Read the model definition and answer for the solid it produces. Units are mm, in the model's axes. Face numbers are marked on the shaded views. A direction names the side the tool comes from. Coordinates: 2 decimals unless noted, no trailing zeros. Write each loop counter-clockwise with the first axis right and the second up, starting at its lowest first coordinate (ties: lowest second). Pieces come first, ordered by that corner, then holes.
(1) Find the intervals of material crossed by probe 1 along Z at (x, y) = (-47.5, -14.5); probe 2 along Z at (x, y) = (-7, -13.5); probe 3 along X at (y, z) = (-8.75, 15), in increasing order.
(2) Which of the six approach directions +Z, -Z, +X, -X, +Y, -Y give full straight-line access (tool end or side, diameter ignored) to the marked faces 5 and 6?
(3) Given pin 1 (6 mm diameter, centred on y = -20.5, z = -2.5, fed in from -X); pin 2 (1 mm diameter, centred on y = -7, z = 52, fed in from +X); pin 3 (1 mm diameter, centred on y = -3.5, z = 47.5, fed in from +X), each flat-ended and moving along its own axis, determine where each tip first touches the part or whether it passes through.
(4) The mould has two halves that part along Z. Classify the marked faces 1, 2, 3 and 4: +Z half, -Z half, draft (parallel to the pull), parting line (faces both ways), or undercut.
(5) Section B-B on y = -13.5 is taken. Write down the section's boundary in (x, z), then the cut area to 3 significant figures.
(6) Section A-A on x = -51.5 is taken. Write down the section's boundary in (y, z), then the cut area to 3 significant figures.
(7) Section D-D on z = 28 is taken. Write down the section's boundary in (x, y).
(8) Section C-C on x = -22.5 is taken. Write down the section's boundary in (y, z).
from build123d import *

# Parameters (mm, degrees)
F1_DEPTH = 25.4


with BuildPart() as f1:
    # F0 (on Front) → F1 (new body)
    with BuildSketch(Plane.XZ):
        with BuildLine():
            Line((6.587991, 76.630748), (-56.699019, 76.630748))
            Line((-56.699019, 76.630748), (-56.699019, 33.66233))
            Line((-56.699019, 33.66233), (-44.595942, 33.66233))
            Line((-44.595942, 33.66233), (-44.595942, -7.400833))
            Line((-44.595942, -7.400833), (-56.699019, -7.400833))
            Line((-56.699019, -7.400833), (-56.699019, -50.369252))
            Line((-56.699019, -50.369252), (6.587991, -50.369252))
            Line((6.587991, -50.369252), (6.587991, -31.048073))
            ThreePointArc((6.587991, -31.048073), (-37.59083, 13.130748), (6.587991, 57.30957))
            Line((6.587991, 57.30957), (6.587991, 76.630748))
        make_face()
    extrude(amount=F1_DEPTH)


solid = f1.part
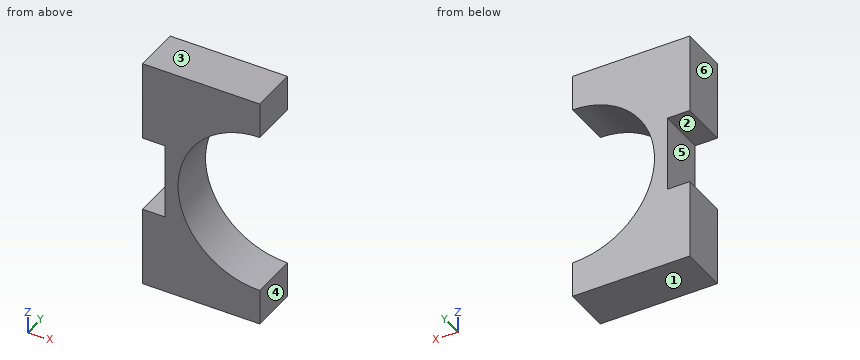
Response:
1. probe 1: z = -50.37 to -7.4, 33.66 to 76.63
1. probe 2: z = -50.37 to -28.91, 55.17 to 76.63
1. probe 3: x = -44.6 to -37.55
2. face 5: -X, +Y, -Y
2. face 6: +Z, -Z, -X, +Y, -Y
3. pin 1: stops at x = -44.6
3. pin 2: stops at x = -13.46
3. pin 3: stops at x = -20.54
4. face 1: -Z half
4. face 2: undercut
4. face 3: +Z half
4. face 4: draft
5. outline: (-56.7, -50.37) - (6.59, -50.37) - (6.59, -31.05) arc R44.18 cw to (6.59, 57.31) - (6.59, 76.63) - (-56.7, 76.63) - (-56.7, 33.66) - (-44.6, 33.66) - (-44.6, -7.4) - (-56.7, -7.4) - close
5. area: 4,470 mm2
6. outline: (-25.4, -50.37) - (0, -50.37) - (0, -7.4) - (-25.4, -7.4) - close; (-25.4, 33.66) - (0, 33.66) - (0, 76.63) - (-25.4, 76.63) - close
6. area: 2,180 mm2
7. outline: (-44.6, -25.4) - (-35.01, -25.4) - (-35.01, 0) - (-44.6, 0) - close
8. outline: (-25.4, -50.37) - (0, -50.37) - (0, -20.12) - (-25.4, -20.12) - close; (-25.4, 46.38) - (0, 46.38) - (0, 76.63) - (-25.4, 76.63) - close
